Input: dimensioned drawing with shaded views. Units: mm. Origin: part minimum x, y, z. A direction names the side the tool comes from. Coordinates: 2 decimals unless noted, no trailing zeros. Loops run counter-clockwise (first coordinate to the right, second up) from the corner with the lowest first, then second, coordinate; pieces in that order, holes last.
Item 1: Section C-C on y = 4. Return loops of the section in (x, z), and give its area (3 significant figures).
Item 2: Reachability of the marked faces 5 and 6 from +Z, -Z, +X, -X, +Y, -Y: full face, straight path, thin tool, end or side. Return the list, or none.
Item 3: Section B-B on z = 3.75. Return loops of the section in (x, y), and give its area (3 significant figures).
Item 4: Pull-direction query (X, two-part tool) for the marked faces 1, 2, 3 and 4; classes: released by +X, released by -X, zero draft, split by the parting line, or undercut.
Item 5: Ray query, line 1 along X through (y, z) = (1.5, 4.75); line 2 along X through (y, z) = (0.45, 3.75); line 3 along Y through (x, z) = (1.75, 5.5). Return the intervals inside material, ascending.
Item 6: Contact query for flat-ended pins moving along their axis: P1, Ø1.5, axis at x = 6.5, y = 5.5, coming from the +Z side; P2, Ø2, axis at x = 3.75, z = 3.75, coming from the -Y side; P3, Ø3.5, axis at x = 3.5, z = 3, coming from the +Y side; P4, Ø3, axis at x = 3.5, y = 4.5, coming from the +Z side. Output: stop coordinate, or through.
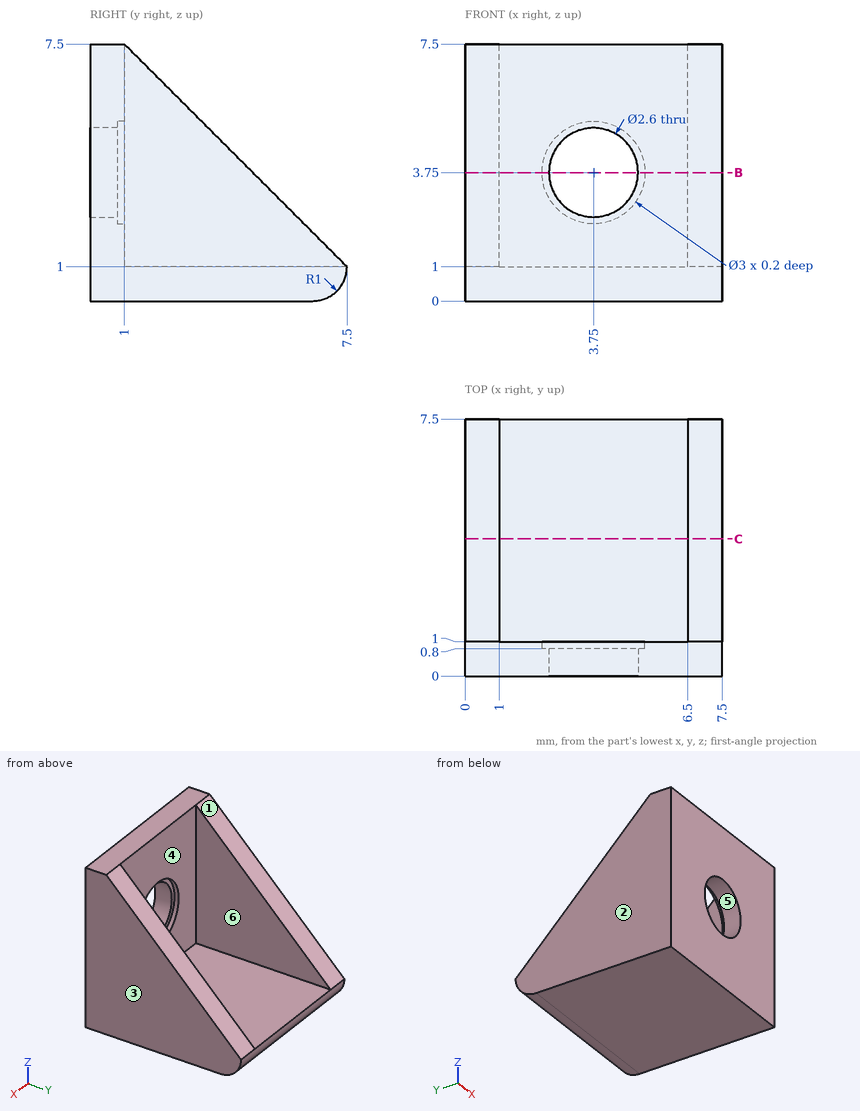
Results found:
1. outline: (0, 0) - (7.5, 0) - (7.5, 4.5) - (6.5, 4.5) - (6.5, 1) - (1, 1) - (1, 4.5) - (0, 4.5) - close
1. area: 14.5 mm2
2. face 5: +Y, -Y
2. face 6: +Z, +Y
3. outline: (0, 0) - (2.45, 0) - (2.45, 0.8) - (2.25, 0.8) - (2.25, 1) - (1, 1) - (1, 4.75) - (0, 4.75) - close; (5.05, 0) - (7.5, 0) - (7.5, 4.75) - (6.5, 4.75) - (6.5, 1) - (5.25, 1) - (5.25, 0.8) - (5.05, 0.8) - close
3. area: 12.3 mm2
4. face 1: zero draft
4. face 2: released by -X
4. face 3: released by +X
4. face 4: undercut
5. line 1: x = 0 to 1, 6.5 to 7.5
5. line 2: x = 0 to 2.45, 5.05 to 7.5
5. line 3: y = 0 to 1
6. P1: stops at z = 3.75
6. P2: passes through
6. P3: stops at y = 1
6. P4: stops at z = 1
